Design review of the part built by this model. Coordinates are the model's own, in mm. Face numbers are marked on the shaded views. A direction names the side the tool comes from. Give positions to 0.01 mm unless a question says otherwise; leave off trailing zeros. Write each loop counter-clockwise with the first axis right and the second up, starting at its lowest first coordinate (ties: lowest second). Pieces come first, ordered by that corner, then holes.
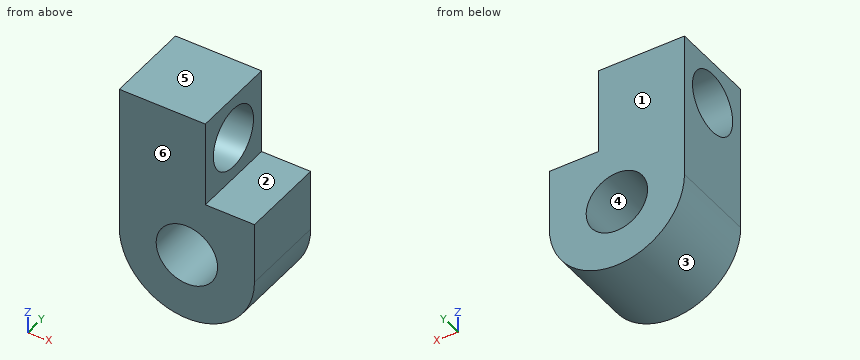
```python
from build123d import *

# Parameters (mm, degrees)
CROQUIS1_R              = 2.5
SALIENTE_EXTRUIR1_DEPTH = 7
CROQUIS3_R              = 2.5
CORTAR_EXTRUIR1_DEPTH   = 17


with BuildPart() as part:
    # Croquis1 → Saliente-Extruir1 (new body)
    with BuildSketch(Plane(origin=(0, 0, 0), x_dir=(1, 0, 0), z_dir=(0, 1, 0))):
        with BuildLine():
            Line((-5.5, 0), (-5.5, -12))
            Line((-5.5, -12), (1.5, -12))
            Line((1.5, -12), (1.5, -5))
            Line((1.5, -5), (5.5, -5))
            Line((5.5, -5), (5.5, 0))
            ThreePointArc((5.5, 0), (0, 5.5), (-5.5, 0))
        make_face()
        with Locations(Location((0, 0, 0), (0, 0, 270))):
            Circle(CROQUIS1_R, mode=Mode.SUBTRACT)
    extrude(amount=SALIENTE_EXTRUIR1_DEPTH)

    # Croquis3 → Cortar-Extruir1 (cut)
    with BuildSketch(Plane.ZY.offset(5.5)):
        with Locations((8.5, 3.5)):
            Circle(CROQUIS3_R)
    extrude(amount=-CORTAR_EXTRUIR1_DEPTH, mode=Mode.SUBTRACT)


solid = part.part
```
(1) Consider section B-B, the plane y = 3.5. Give the boundary of the cut face in (x, z).
Resolved:
outline: (-5.5, 0) arc R5.5 ccw to (5.5, 0) - (5.5, 5) - (1.5, 5) - (1.5, 6) - (-5.5, 6) - close; (-5.5, 11) - (1.5, 11) - (1.5, 12) - (-5.5, 12) - close; hole circle Ø5 at (0, 0)
(2) Consider section D-D, the plane y = 2. Give the boundary of the cut face in (x, z).
Resolved:
outline: (-5.5, 0) arc R5.5 ccw to (5.5, 0) - (5.5, 5) - (1.5, 5) - (1.5, 6.5) - (-5.5, 6.5) - close; (-5.5, 10.5) - (1.5, 10.5) - (1.5, 12) - (-5.5, 12) - close; hole circle Ø5 at (0, 0)
(3) Consider section C-C, the plane z = 8.5. Give the boundary of the cut face in (x, y), then the cut area to 3 significant figures.
Resolved:
outline: (-5.5, 0) - (1.5, 0) - (1.5, 1) - (-5.5, 1) - close; (-5.5, 6) - (1.5, 6) - (1.5, 7) - (-5.5, 7) - close
area: 14.0 mm2
(4) Mouldability with a two-part tool opening along Z and no side actions: class the marked faces 3, 4, 5 and 6 as pulls with the +Z half, pulls with the -Z half, needs draft (parallel to the pull), parting line crosses it, or undercut.
Resolved:
face 3: pulls with the -Z half
face 4: undercut
face 5: pulls with the +Z half
face 6: needs draft
(5) Tool access review of the marked faces 1 and 2: name each direction out of +Z, -Z, +X, -X, +Y, -Y from which nothing blocks a thin tool from reaching the whole face with its end or side.
Resolved:
face 1: +Z, -Z, +X, -X, +Y
face 2: +Z, +X, +Y, -Y
(6) Clearance check with flat-ended pins moving along their axes: P1, Ø6, axis at x = -2.5, z = 8, coming from the -Y side; P2, Ø2, axis at x = 3.5, y = 2, coming from the +Z side; P3, Ø4, axis at x = 4, y = 1.5, coming from the -Z side; P4, Ø4.5, axis at x = 0, z = 0, coming from the -Y side. State where each tip first meets the part, or that it passes through.
Resolved:
P1: stops at y = 0
P2: stops at z = 5
P3: stops at z = -5.12
P4: passes through
(7) To check wall thickness, follow L1, parallel to Y at x = -2, z = 8.5; L2, parallel to Z at x = -1.75, y = 2.5; L3, parallel to Z at x = -0.75, y = 4. State the ranges of each line that lie inside material, in increasing order.
Resolved:
L1: y = 0 to 1, 6 to 7
L2: z = -5.21 to -1.79, 1.79 to 6.21, 10.79 to 12
L3: z = -5.45 to -2.38, 2.38 to 6.05, 10.95 to 12
(8) Consider section A-A, the plane x = 0. Give the boundary of the cut face in (y, z), then the cut area to 3 significant figures.
Resolved:
outline: (0, -5.5) - (7, -5.5) - (7, -2.5) - (0, -2.5) - close; (0, 2.5) - (7, 2.5) - (7, 12) - (0, 12) - close; hole circle Ø5 at (3.5, 8.5)
area: 67.9 mm2
